Verification items for this drawing (mm, ordinates from the low corner). Give positions to 0.01 mm unless a question says otherwise; leave off trailing zeros. Order: outer loops, then holes, each group sorted by start corner. A loop starts at its lowest first (then second) coordinate and runs counter-clockwise, first axis right, second up.
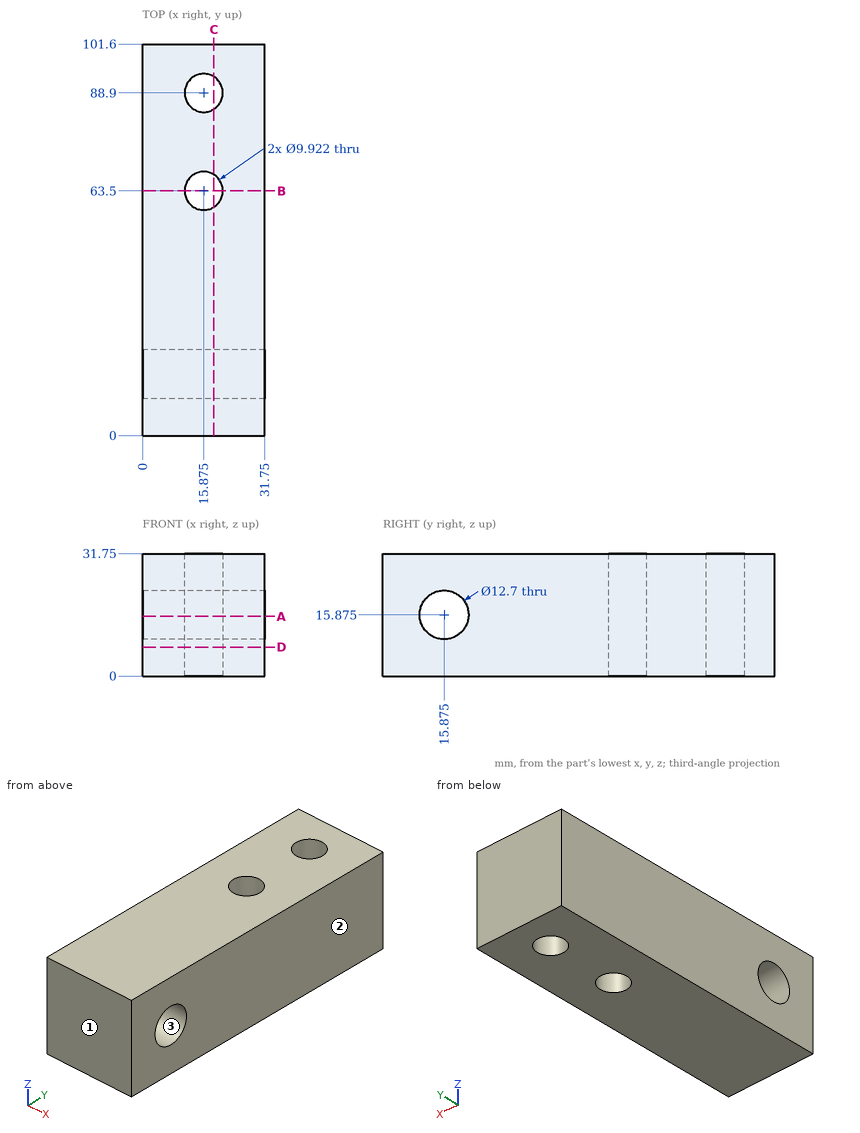
Q1. Thickness scan on L1, parallel to Y at x = 14.5, z = 6.5; L2, parallel to Y at x = 14, z = 13; L3, parallel to Y at x = 12, z = 11. Record the ranges inside material, lowest first.
Q2. Cross-section at C-C, the plane x = 18.5. Give the number of separate pieces and of enclosed holes in the cut face, and give its area (3 significant figures).
Q3. Cross-section at A-A, the plane z = 15.5. Record the boundary of the cut face in (x, y) (3 decimals).
Q4. Release check for a two-part mould opening along Y. For the marked faces 1, 2 and 3 record: pulls with the +Y half, pulls with the -Y half, needs draft (parallel to the pull), parting line crosses it, or undercut.
Q5. Cross-section at B-B, the plane y = 63.5. Record the boundary of the cut face in (x, z).
Q6. Cross-section at D-D, the plane z = 7.5. Record the boundary of the cut face in (x, y) (3 decimals), and give its area (3 significant figures).
Q7. Gauge pin test, flat end, axial feed: P1, Ø10, axis at x = 25.5, z = 12, coming from the -Y side. Record the tip position at first contact, or that the pin passes through.
Answers follow:
1. L1: y = 0 to 58.73, 68.27 to 84.13, 93.67 to 101.6
1. L2: y = 0 to 10.21, 21.54 to 58.91, 68.09 to 84.31, 93.49 to 101.6
1. L3: y = 0 to 11.81, 19.94 to 60.4, 66.6 to 85.8, 92 to 101.6
2. separate pieces: 3
2. enclosed holes: 1
2. area: 2,560 mm2
3. outline: (0, 0) - (31.75, 0) - (31.75, 9.536) - (0, 9.536) - close; (0, 22.214) - (31.75, 22.214) - (31.75, 101.6) - (0, 101.6) - close; hole circle Ø9.922 at (15.875, 63.5); hole circle Ø9.922 at (15.875, 88.9)
4. face 1: pulls with the -Y half
4. face 2: needs draft
4. face 3: undercut
5. outline: (0, 0) - (10.91, 0) - (10.91, 31.75) - (0, 31.75) - close; (20.84, 0) - (31.75, 0) - (31.75, 31.75) - (20.84, 31.75) - close
6. outline: (0, 0) - (31.75, 0) - (31.75, 101.6) - (0, 101.6) - close; hole circle Ø9.922 at (15.875, 63.5); hole circle Ø9.922 at (15.875, 88.9)
6. area: 3,070 mm2
7. P1: stops at y = 0
